Read the model definition and answer for the solid it produces. Units are mm, in the model's axes. Round coordinates to 2 decimals unless told otherwise and drop trailing zeros. Write each loop counter-clockwise with the first axis right and the second up, starting at its lowest first coordinate (ties: lowest second). Pieces come first, ordered by that corner, then holes. Notation, with made-up numbers: (67.5, 82.25) - (86.5, 82.25) arc R22 ccw to (86.5, 121.25) - close; hole circle Ø9 at (9, 16.25). An arc over 180 degrees is marked (long way). Answer as CSV lines item,"result". Start each with the question number.
1) Find section C-C on z = 6.5. Determine the outline of the cut face in (x, y), then the cut area to 3 significant figures.
2) Find section A-A on x = 38.5. Determine the outline of the cut face in (y, z), then the cut area to 3 significant figures.
3) Each of these flat-tipped pins is pushed along its axis until it touches: pin 1 (1.6 mm diameter, centred on x = -36.5, y = 0.5, fed in from -Z); pin 2 (1 mm diameter, centred on y = 0, z = 25, fed in from +X). Where does it stop, or does it pass through?
4) Find section B-B on x = -80. Determine the outline of the cut face in (y, z).
5) Consider line 1 along Z through (x, y) = (24, -0.85); line 2 along Z through (x, y) = (32.5, 1.45); line 3 along X through (y, z) = (-1.3, -52). Determine where each line is inside the solid, lowest interval first.
from build123d import *

# Parameters (mm, degrees)
BOSS_EXTRUDE1_DEPTH = 1.5875
CUT_EXTRUDE1_DEPTH  = 152.481733807


with BuildPart() as part:
    # Sketch1 → Boss-Extrude1 (new, symmetric)
    with BuildSketch(Plane(origin=(0, 0, 0), x_dir=(1, 0, 0), z_dir=(0, 1, 0))):
        Polygon((-122.014602546, 89.716619519), (-71.214602546, 89.716619519), (-71.214602546, 86.541619519), (-58.514602546, 86.541619519), (-58.514602546, 89.716619519), (-45.814602546, 89.716619519), (-45.814602546, 86.541619519), (-33.114602546, 86.541619519), (-33.114602546, 89.716619519), (-20.414602546, 89.716619519), (-20.414602546, 86.541619519), (-7.714602546, 86.541619519), (-7.714602546, 89.716619519), (4.985397454, 89.716619519), (4.985397454, 86.541619519), (17.685397454, 86.541619519), (17.685397454, 89.716619519), (30.385397454, 89.716619519), (30.385397454, 86.541619519), (43.085397454, 86.541619519), (43.085397454, 89.716619519), (93.885397454, 89.716619519), (93.885397454, 54.791619519), (90.710397454, 54.791619519), (90.710397454, 42.091619519), (93.885397454, 42.091619519), (93.885397454, 29.391619519), (90.710397454, 29.391619519), (90.710397454, 16.691619519), (93.885397454, 16.691619519), (93.885397454, 3.991619519), (90.710397454, 3.991619519), (90.710397454, -8.708380481), (93.885397454, -8.708380481), (93.885397454, -21.408380481), (90.710397454, -21.408380481), (90.710397454, -34.108380481), (93.885397454, -34.108380481), (93.885397454, -69.033380481), (43.085397454, -69.033380481), (43.085397454, -65.858380481), (30.385397454, -65.858380481), (30.385397454, -69.033380481), (17.685397454, -69.033380481), (17.685397454, -65.858380481), (4.985397454, -65.858380481), (4.985397454, -69.033380481), (-7.714602546, -69.033380481), (-7.714602546, -65.858380481), (-20.414602546, -65.858380481), (-20.414602546, -69.033380481), (-33.114602546, -69.033380481), (-33.114602546, -65.858380481), (-45.814602546, -65.858380481), (-45.814602546, -69.033380481), (-58.514602546, -69.033380481), (-58.514602546, -65.858380481), (-71.214602546, -65.858380481), (-71.214602546, -69.033380481), (-122.014602546, -69.033380481), (-122.014602546, -34.108380481), (-118.839602546, -34.108380481), (-118.839602546, -21.408380481), (-122.014602546, -21.408380481), (-122.014602546, -8.708380481), (-118.839602546, -8.708380481), (-118.839602546, 3.991619519), (-122.014602546, 3.991619519), (-122.014602546, 16.691619519), (-118.839602546, 16.691619519), (-118.839602546, 29.391619519), (-122.014602546, 29.391619519), (-122.014602546, 42.091619519), (-118.839602546, 42.091619519), (-118.839602546, 54.791619519), (-122.014602546, 54.791619519), align=None)
    extrude(amount=BOSS_EXTRUDE1_DEPTH, both=True)

    # Sketch2 → Cut-Extrude1 (cut, through all)
    with BuildSketch(Plane(origin=(0, 1.5875, 0), x_dir=(1, 0, 0), z_dir=(0, 1, 0))):
        with BuildLine():
            Line((81.185397454, 6.531619519), (-109.314602546, 6.531619519))
            ThreePointArc((-109.314602546, 6.531619519), (-113.124602546, 10.341619519), (-109.314602546, 14.151619519))
            Line((-109.314602546, 14.151619519), (81.185397454, 14.151619519))
            ThreePointArc((81.185397454, 14.151619519), (84.995397454, 10.341619519), (81.185397454, 6.531619519))
        make_face()
    extrude(amount=-CUT_EXTRUDE1_DEPTH, mode=Mode.SUBTRACT)


solid = part.part
Check values:
1,outline,"(-118.84, -1.59) - (90.71, -1.59) - (90.71, 1.59) - (-118.84, 1.59) - close"
1,area,"665 mm^2"
2,outline,"(-1.59, -86.54) - (1.59, -86.54) - (1.59, -14.15) - (-1.59, -14.15) - close; (-1.59, -6.53) - (1.59, -6.53) - (1.59, 65.86) - (-1.59, 65.86) - close"
2,area,"460 mm^2"
3,pin 1,"stops at z = -86.54"
3,pin 2,"stops at x = 90.71"
4,outline,"(-1.59, -89.72) - (1.59, -89.72) - (1.59, -14.15) - (-1.59, -14.15) - close; (-1.59, -6.53) - (1.59, -6.53) - (1.59, 69.03) - (-1.59, 69.03) - close"
5,line 1,"z = -89.72 to -14.15, -6.53 to 69.03"
5,line 2,"z = -86.54 to -14.15, -6.53 to 65.86"
5,line 3,"x = -118.84 to 90.71"
